For this review, use the dimensioned drawing (mm, ordinates from the lowest corner) and the shaded views. A direction names the side the tool comes from. Round coordinates to 2 decimals unless told otherwise and drop trailing zeros. Loops run counter-clockwise (first coordinate to the right, second up) from the corner with the lowest first, then second, coordinate; pieces in that order, holes last. Notation, with made-up numbers: M 71.25,61.5 L 112.25,61.5 A22 cw 112.25,85.5 Z; hole C 19.25,80.25 d1. An arc over 180 degrees is marked long. One line per item, written item: value. Start each with the question number.
Item 1: For line 1 along Z through (x, y) = (1.3, 8); line 2 along Y through (x, z) = (7.75, 23.5); line 3 along Y through (x, z) = (3.6, 28.5), list the stretches that pass through material, from the lowest coordinate up.
Item 2: For the marked faces 1, 2 and 3, list the 3-axis set-ups (+Z, -Z, +X, -X, +Y, -Y) from which the entire face can be reached by the end or side of a thin tool; tool diameter is ignored.
Item 3: Mouldability with a two-part tool opening along X and no side actions: class the marked faces 4, 5 and 6 as released by +X, released by -X, zero draft, split by the parting line, or undercut.
Item 4: We need section A-A (y = 8). State how many separate pieces and enclosed holes the cut face has, then the cut area to 3 significant figures.
Item 5: We need section D-D (z = 22.5). Write out the cut boundary in (x, y), then the cut area to 3 significant figures.
Item 6: We need section B-B (z = 15.5). Write out the cut boundary in (x, y).
Item 7: Clearance check with flat-ended pins moving along their axes: pin 1 (5 mm diameter, centred on x = 8, y = 8, fed in from +Z); pin 2 (6 mm diameter, centred on y = 13, z = 28, fed in from -X); pin 3 (3 mm diameter, centred on y = 5.5, z = 15.5, fed in from +X); pin 4 (5 mm diameter, centred on x = 14, z = 26, fed in from -Y). State where each tip first meets the part, or that it passes through.
Item 8: We need section C-C (z = 28.5). Write out the cut boundary in (x, y) (3 decimals).
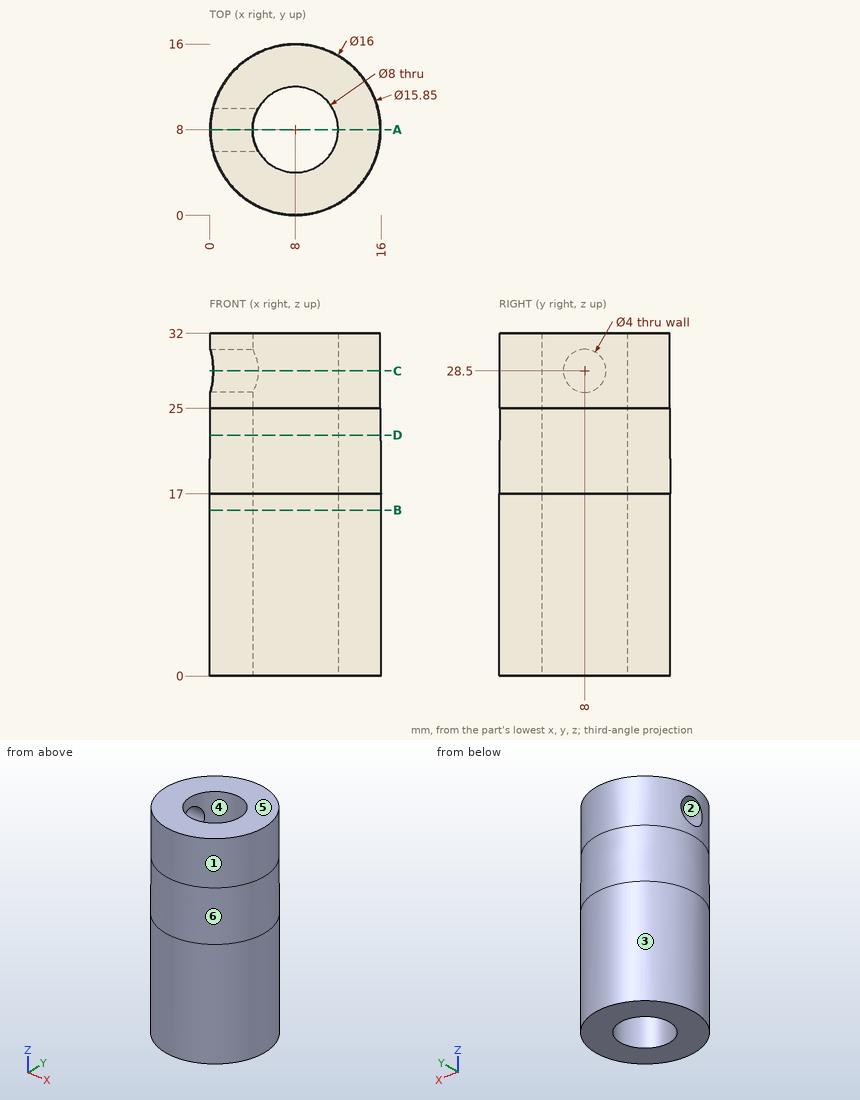
A:
1. line 1: 0 to 26.5, 30.5 to 32
1. line 2: 0.06 to 4.01, 11.99 to 15.94
1. line 3: 1.41 to 6, 10 to 14.59
2. face 1: +Z
2. face 2: -X
2. face 3: +Z, -Z
3. face 4: undercut
3. face 5: zero draft
3. face 6: split by the parting line
4. separate pieces: 3
4. enclosed holes: 0
4. area: 239 mm2
5. outline: C 8,8 d15.9; hole C 8,8 d8
5. area: 148 mm2
6. outline: C 8,8 d16; hole C 8,8 d8
7. pin 1: through
7. pin 2: x = 0.33
7. pin 3: x = 15.94
7. pin 4: y = 0.89
8. outline: M 0.332,6 A7.925 ccw long 0.332,10 L 4.536,10 A4 cw long 4.536,6 Z
